from build123d import *

# Parameters (mm, degrees)
SKETCH_1_R          = 29.5
EXTRUDE_1_DEPTH     = 4
SKETCH_2_W          = 28.166253132
SKETCH_2_H          = 32.95394871
CUT_EXTRUDE_1_DEPTH = 42.910619179
SKETCH_3_W          = 38
SKETCH_3_H          = 7.946399408
CUT_EXTRUDE_2_DEPTH = 40.47360569
SKETCH_6_R          = 1.6
CUT_EXTRUDE_5_DEPTH = 40.47360569


with BuildPart() as part:
    # 草图1 → 凸台-拉伸1 (new body)
    with BuildSketch(Plane(origin=(0, 0, 0), x_dir=(1, 0, 0), z_dir=(0, 1, 0))):
        with Locations(Location((0, 0, 0), (0, 0, 270))):
            Circle(SKETCH_1_R)
    extrude(amount=EXTRUDE_1_DEPTH)

    # 草图2 → 切除-拉伸1 (cut, through all)
    with BuildSketch(Plane(origin=(0, 4, 0), x_dir=(1, 0, 0), z_dir=(0, 1, 0))):
        with Locations((0, 29.5)):
            Rectangle(SKETCH_2_W, SKETCH_2_H)
        with Locations((0, -29.5)):
            Rectangle(SKETCH_2_W, SKETCH_2_H)
    extrude(amount=-CUT_EXTRUDE_1_DEPTH, mode=Mode.SUBTRACT)

    # 草图3 → 切除-拉伸2 (cut, through all)
    with BuildSketch(Plane(origin=(0, 4, 0), x_dir=(1, 0, 0), z_dir=(0, 1, 0))):
        Rectangle(SKETCH_3_W, SKETCH_3_H)
    extrude(amount=-CUT_EXTRUDE_2_DEPTH, mode=Mode.SUBTRACT)

    # 草图6 → 切除-拉伸5 (cut, through all)
    with BuildSketch(Plane(origin=(0, 4, 0), x_dir=(1, 0, 0), z_dir=(0, 1, 0))):
        with Locations(Location((-25.893583016, 0, 0), (0, 0, 270))):
            Circle(SKETCH_6_R)
        with Locations(Location((26.106416984, 0, 0), (0, 0, 270))):
            Circle(SKETCH_6_R)
        with Locations(Location((-21.376, 12.613, 0), (0, 0, 270))):
            Circle(SKETCH_6_R)
        with Locations(Location((21.376, 12.613, 0), (0, 0, 270))):
            Circle(SKETCH_6_R)
        with Locations(Location((-21.376, -12.613, 0), (0, 0, 270))):
            Circle(SKETCH_6_R)
        with Locations(Location((21.376, -12.613, 0), (0, 0, 270))):
            Circle(SKETCH_6_R)
    extrude(amount=-CUT_EXTRUDE_5_DEPTH, mode=Mode.SUBTRACT)


solid = part.part
Geometry: final body of the model. Coordinates: model frame, mm. A direction names the side the tool comes from. Round coordinates to 2 decimals unless told otherwise and drop trailing zeros. Order: outer loops, then holes, each group sorted by start corner. A loop starts at its lowest first (then second) coordinate and runs counter-clockwise, first axis right, second up.
Q1. Section C-C, the plane y = 1.95. Output: boundary loops of the cut face in (x, z).
Result sheet:
outline: (-14.08, -25.92) - (-14.08, -13.02) - (14.08, -13.02) - (14.08, -25.92) arc R29.5 ccw to (14.08, 25.92) - (14.08, 13.02) - (-14.08, 13.02) - (-14.08, 25.92) arc R29.5 ccw to start; hole circle Ø3.2 at (-25.89, 0); hole circle Ø3.2 at (-21.38, -12.61); hole circle Ø3.2 at (-21.38, 12.61); hole (-19, -3.97) - (19, -3.97) - (19, 3.97) - (-19, 3.97) - close; hole circle Ø3.2 at (21.38, -12.61); hole circle Ø3.2 at (21.38, 12.61); hole circle Ø3.2 at (26.11, 0)
Q2. Pin query (flat end, axial travel): pin 1 (2 mm diameter, centred on y = 2, z = 17.5, fed in from -X); pin 2 (1 mm diameter, centred on x = -21.5, y = 2, fed in from -Z); pin 3 (2 mm diameter, centred on y = 2, z = -19.5, fed in from -X); pin 4 (1.9 mm diameter, centred on x = 21.376, z = -12.613, fed in from +Y). Return the tip coordinate at first contact, or that it passes through.
Result sheet:
pin 1: stops at x = -24.45
pin 2: stops at z = -20.72
pin 3: stops at x = -22.98
pin 4: passes through
Q3. Mould query, pull axis X, two halves, no side actions, for faces 4 (the face through (29.497, 1.972, 0.443)), 5 (the face through (0, 0, 5)), 6 (the face through (14.083, 2, 20)), 7 (the face through (-29.497, 1.972, -0.443)). Classes: released by +X, released by -X, zero draft, split by the parting line, or undercut.
Result sheet:
face 4: released by +X
face 5: zero draft
face 6: undercut
face 7: released by -X
Q4. Material intervals for probe 1 along Z at (x, y) = (-5, 0.3); probe 2 along Z at (x, y) = (22.5, 2.9); probe 3 along X at (y, z) = (3.15, -13.5), sorted ascending.
Result sheet:
probe 1: z = -13.02 to -3.97, 3.97 to 13.02
probe 2: z = -19.08 to -13.75, -11.47 to 11.47, 13.75 to 19.08
probe 3: x = -26.23 to -22.71, -20.04 to -14.08, 14.08 to 20.04, 22.71 to 26.23
Q5. Access query for faces 1 (the face through (-14.083, 2, 20)), 2 (the face through (-19, 2, 0)), 3 (the face through (14.083, 2, -19)). Directions: +Z, -Z, +X, -X, +Y, -Y. A direction counts if a zero-diameter tool reaches every point of the face in a straight line with its end or side. Return the directions, or none.
Result sheet:
face 1: +Z, +Y, -Y
face 2: +Y, -Y
face 3: -Z, +Y, -Y
Q6. Section B-B, the plane z = 0. Output: boundary loops of the cut face in (x, y), and give its area (3 significant figures).
Result sheet:
outline: (-29.5, 0) - (-27.49, 0) - (-27.49, 4) - (-29.5, 4) - close; (-24.29, 0) - (-19, 0) - (-19, 4) - (-24.29, 4) - close; (19, 0) - (24.51, 0) - (24.51, 4) - (19, 4) - close; (27.71, 0) - (29.5, 0) - (29.5, 4) - (27.71, 4) - close
area: 58.4 mm2
Q7. Section A-A, the plane x = -1. Output: boundary loops of the cut face in (y, z), and give its area (3 significant figures).
Result sheet:
outline: (0, -13.02) - (4, -13.02) - (4, -3.97) - (0, -3.97) - close; (0, 3.97) - (4, 3.97) - (4, 13.02) - (0, 13.02) - close
area: 72.4 mm2
Q8. Section D-D, the plane z = -7. Output: boundary loops of the cut face in (x, y), and give its area (3 significant figures).
Result sheet:
outline: (-28.66, 0) - (28.66, 0) - (28.66, 4) - (-28.66, 4) - close
area: 229 mm2
